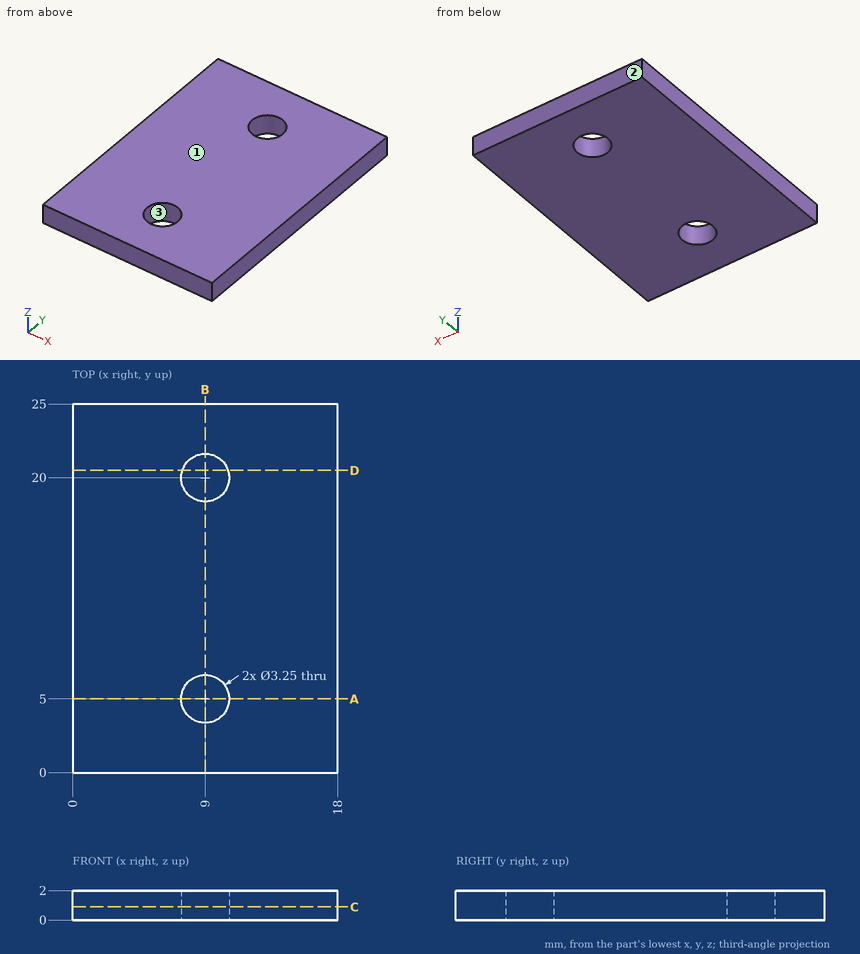
For this review, use the dimensioned drawing (mm, ordinates from the lowest corner) and the shaded views. Give positions to 0.01 mm unless a question says otherwise; leave off trailing zeros. Order: outer loops, then holes, each group sorted by start corner. A loop starts at its lowest first (then second) coordinate and runs counter-clockwise, first axis right, second up.
1) Take a section at D-D (y = 20.5). Give the boundary of the cut face in (x, z).
2) Take a section at A-A (y = 5). Give the boundary of the cut face in (x, z) (3 decimals), then the cut area to 3 significant figures.
3) Take a section at C-C (z = 0.9). Give the boundary of the cut face in (x, y) (3 decimals).
4) Take a section at B-B (x = 9). Give the boundary of the cut face in (y, z) (3 decimals), then the cut area to 3 significant figures.
5) Wall thickness on line 1 (Y direction, x = 9, z = 0.6) (3 decimals); line 2 (X direction, y = 5, z = 0.5) (3 decimals); line 3 (Y direction, x = 10, z = 0.75): over which ranges is each line inside the solid? List them lowest first.
6) The part is to be moulded in two halves that separate along Y. For the marked faces 1, 2 and 3, say which applies: released by +Y, released by -Y, zero draft, split by the parting line, or undercut.
Derived:
1. outline: (0, 0) - (7.45, 0) - (7.45, 2) - (0, 2) - close; (10.55, 0) - (18, 0) - (18, 2) - (10.55, 2) - close
2. outline: (0, 0) - (7.375, 0) - (7.375, 2) - (0, 2) - close; (10.625, 0) - (18, 0) - (18, 2) - (10.625, 2) - close
2. area: 29.5 mm2
3. outline: (0, 0) - (18, 0) - (18, 25) - (0, 25) - close; hole circle Ø3.25 at (9, 5); hole circle Ø3.25 at (9, 20)
4. outline: (0, 0) - (3.375, 0) - (3.375, 2) - (0, 2) - close; (6.625, 0) - (18.375, 0) - (18.375, 2) - (6.625, 2) - close; (21.625, 0) - (25, 0) - (25, 2) - (21.625, 2) - close
4. area: 37.0 mm2
5. line 1: y = 0 to 3.375, 6.625 to 18.375, 21.625 to 25
5. line 2: x = 0 to 7.375, 10.625 to 18
5. line 3: y = 0 to 3.72, 6.28 to 18.72, 21.28 to 25
6. face 1: zero draft
6. face 2: released by +Y
6. face 3: undercut
